from build123d import *

# Parameters (mm, degrees)
SKETCH1_R           = 15
SKETCH1_R_2         = 12
BOSS_EXTRUDE1_DEPTH = 22
BOSS_EXTRUDE3_DEPTH = 16
SKETCH9_W           = 75.776541305
SKETCH9_H           = 5
CUT_EXTRUDE1_DEPTH  = 42
SKETCH10_W          = 75.776541305
SKETCH10_H          = 5
CUT_EXTRUDE2_DEPTH  = 42


with BuildPart() as part:
    # Sketch1 → Boss-Extrude1 (new body)
    with BuildSketch(Plane.XY):
        with BuildLine():
            Line((55.604384426, -9.406151738), (55.604384426, -41.038199431))
            ThreePointArc((55.604384426, -41.038199431), (53.847025113, -45.280840118), (49.604384426, -47.038199431))
            Line((49.604384426, -47.038199431), (5.604384426, -47.038199431))
            ThreePointArc((5.604384426, -47.038199431), (1.361743739, -45.280840118), (-0.395615574, -41.038199431))
            Line((-0.395615574, -41.038199431), (-0.395615574, -13.257389991))
            ThreePointArc((-0.395615574, -13.257389991), (-2.152974887, -9.014749304), (-6.395615574, -7.257389991))
            Line((-6.395615574, -7.257389991), (-51.162903124, -7.257389991))
            Line((-51.162903124, -7.257389991), (-51.162903124, 8.742610009))
            ThreePointArc((-51.162903124, 8.742610009), (-3.834966472, 18.603456094), (37.620760235, 43.474977893))
            ThreePointArc((37.620760235, 43.474977893), (79.465755498, 34.75331261), (60.435706944, -3.5210695))
            ThreePointArc((60.435706944, -3.5210695), (56.966924728, -5.599057366), (55.604384426, -9.406151738))
        make_face()
        with Locations((55.176658278, 22.961800569)):
            Circle(SKETCH1_R, mode=Mode.SUBTRACT)
        with Locations((27.176658278, -27.038199431)):
            Circle(SKETCH1_R_2, mode=Mode.SUBTRACT)
    extrude(amount=BOSS_EXTRUDE1_DEPTH)

    # Sketch7 → Boss-Extrude3 (add)
    with BuildSketch(Plane.XZ.offset(7.257389991)):
        with BuildLine():
            ThreePointArc((-36.240473941, -43.544887573), (-38.141585084, -58.103978296), (-51.162903124, -64.888270652))
            Line((-51.162903124, -64.888270652), (-95.162903124, -64.888270652))
            ThreePointArc((-95.162903124, -64.888270652), (-109.449332837, -55.952342799), (-107.665731017, -39.196100826))
            Line((-107.665731017, -39.196100826), (-74.842207937, 2.663454503))
            ThreePointArc((-74.842207937, 2.663454503), (-72.680751998, 6.589987728), (-71.87991075, 11))
            ThreePointArc((-71.87991075, 11), (-72.680751998, 15.410012272), (-74.842207937, 19.336545497))
            Line((-74.842207937, 19.336545497), (-107.665731017, 61.196100826))
            ThreePointArc((-107.665731017, 61.196100826), (-109.449332837, 77.952342799), (-95.162903124, 86.888270652))
            Line((-95.162903124, 86.888270652), (-51.162903124, 86.888270652))
            ThreePointArc((-51.162903124, 86.888270652), (-38.141585084, 80.103978296), (-36.240473941, 65.544887573))
            ThreePointArc((-36.240473941, 65.544887573), (-32.791035654, 35.909068602), (-6.395615574, 22))
            Line((-6.395615574, 22), (-51.162903124, 22))
            Line((-51.162903124, 22), (-51.162903124, 0))
            Line((-51.162903124, 0), (-6.395615574, 0))
            ThreePointArc((-6.395615574, 0), (-32.791035654, -13.909068602), (-36.240473941, -43.544887573))
        make_face()
        with BuildLine():
            ThreePointArc((-51.162903124, -58.536156571), (-41.626746553, -49), (-51.162903124, -39.463843429))
            Line((-51.162903124, -39.463843429), (-95.162903124, -39.463843429))
            ThreePointArc((-95.162903124, -39.463843429), (-104.699059695, -49), (-95.162903124, -58.536156571))
            Line((-95.162903124, -58.536156571), (-51.162903124, -58.536156571))
        make_face(mode=Mode.SUBTRACT)
        with BuildLine():
            ThreePointArc((-95.162903124, 80.536156571), (-104.699059695, 71), (-95.162903124, 61.463843429))
            Line((-95.162903124, 61.463843429), (-51.162903124, 61.463843429))
            ThreePointArc((-51.162903124, 61.463843429), (-41.626746553, 71), (-51.162903124, 80.536156571))
            Line((-51.162903124, 80.536156571), (-95.162903124, 80.536156571))
        make_face(mode=Mode.SUBTRACT)
    extrude(amount=-BOSS_EXTRUDE3_DEPTH)

    # Sketch9 → Cut-Extrude1 (cut)
    with BuildSketch(Plane.XY.offset(86.888270652)):
        with Locations((-73.162903125, 6.242610009)):
            Rectangle(SKETCH9_W, SKETCH9_H)
    extrude(amount=-CUT_EXTRUDE1_DEPTH, mode=Mode.SUBTRACT)

    # Sketch10 → Cut-Extrude2 (cut)
    with BuildSketch(Plane(origin=(0, 0, -64.888270652), x_dir=(-1, 0, 0), z_dir=(0, 0, -1))):
        with Locations((73.162903125, 6.242610009)):
            Rectangle(SKETCH10_W, SKETCH10_H)
    extrude(amount=-CUT_EXTRUDE2_DEPTH, mode=Mode.SUBTRACT)


solid = part.part
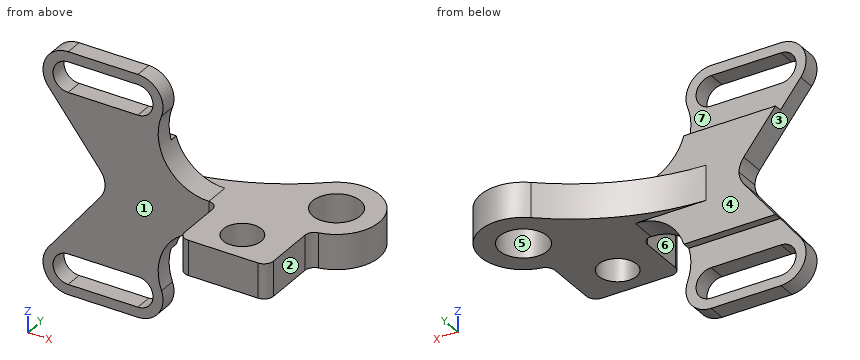
Model file for the job. Use its own axes, mm. Face numbers are marked on the shaded views. A direction names the side the tool comes from. Give positions to 0.01 mm unless a question says otherwise; leave off trailing zeros. Loops run counter-clockwise (first coordinate to the right, second up) from the corner with the lowest first, then second, coordinate; pieces in that order, holes last. Notation, with made-up numbers: (-5.75, -30) - (17.25, -30) arc R32 cw to (17.25, 5) - close; hole circle Ø10 at (13.25, 33.25). An arc over 180 degrees is marked (long way). Use one line per item in the form item = value.
(1) Cut at A-A (z = -49). Give the cut face in (x, y).
Determined:
outline = (-111.05, -7.26) - (-104.7, -7.26) - (-104.7, 3.74) - (-111.05, 3.74) - close; (-41.63, -7.26) - (-35.27, -7.26) - (-35.27, 3.74) - (-41.63, 3.74) - close
(2) Pull direction X, two halves, no side cores. Call the marked faces 5, 6 and 7: pulls with the +X half, pulls with the -X half, needs draft (parallel to the pull), parting line crosses it, or undercut.
Determined:
face_5 = undercut
face_6 = pulls with the -X half
face_7 = needs draft
(3) Cut at C-C (y = 34). Give the cut face in (x, z).
Determined:
outline = (25.26, 0) - (45.02, 0) - (45.02, 22) - (25.26, 22) - close; (65.33, 0) - (79.82, 0) - (79.82, 22) - (65.33, 22) - close
(4) Drill centre lines: L1, parallel to Z at x = -89, y = -2; L2, parallel to Y at x = -61.5, z = 4; L3, parallel to Z at x = 34.5, y = -38. Where is each one in solid material? Low to high.
Determined:
L1 = -64.89 to -58.54, -39.46 to -15.39, 37.39 to 61.46, 80.54 to 86.89
L2 = -7.26 to 8.74
L3 = 0 to 22
(5) Drop flat-ended pins along their axis: P1, Ø11, axis at y = -29, z = 8, coming from the -X side; P2, Ø8, axis at x = 37, y = 7, coming from the +Z side; P3, Ø4, axis at x = -72, y = 6.5, coming from the -Z side. Give the stop position or say it passes through.
Determined:
P1 = -0.4
P2 = 22
P3 = -22.89
(6) Cut at D-D (z = 53). Give the cut face in (x, y), then the cut area to 3 significant figures.
Determined:
outline = (-101.24, -7.26) - (-38.38, -7.26) - (-38.38, 3.74) - (-101.24, 3.74) - close
area = 691 mm^2
(7) 3-axis set-ups, long thin cutter, end or side, ignore diameter. For the marked faces 1, 2, 3 and 4: which of +Z, -Z, +X, -X, +Y, -Y reach the whole face in a straight line?
Determined:
face_1 = +Z, -Z, -X, -Y
face_2 = +Z, -Z, +X, -Y
face_3 = -X, +Y, -Y
face_4 = -X, +Y
(8) Cut at B-B (x = -47). Give the cut face in (y, z), then the cut area to 3 significant figures.
Determined:
outline = (-7.26, -64.33) - (3.74, -64.33) - (3.74, -57.58) - (-7.26, -57.58) - close; (-7.26, -40.42) - (3.74, -40.42) - (3.74, -22.89) - (8.74, -22.89) - (8.74, 0) - (8.96, 0) - (8.96, 22) - (8.74, 22) - (8.74, 44.89) - (3.74, 44.89) - (3.74, 62.42) - (-7.26, 62.42) - close; (-7.26, 79.58) - (3.74, 79.58) - (3.74, 86.33) - (-7.26, 86.33) - close
area = 1,620 mm^2
